The figure shows three views and two pictorial views of one solid part (mm, origin at its lowest corner). Answer the questions. Round coordinates to 2 decimals unless told otherwise and drop trailing zeros. Order: outer loops, then holes, each group sorted by start corner. A loop starts at its lowest first (then second) coordinate and runs counter-clockwise, first axis right, second up. Notation, with made-up numbers: (5, 13.25) - (31, 13.25) arc R33 ccw to (31, 50.25) - close; hole circle Ø7 at (87, 20). An arc over 180 degrees is marked (long way). Answer as a JSON object with one key per item and string values. Group by question number.
Q1. A cutting plane is placed at A-A on x = 10. Determine the outline of the cut face in (y, z), and give its area (3 significant figures).
Q2. A cutting plane is placed at C-C on y = 1. Determine the outline of the cut face in (x, z), and give its area (3 significant figures).
Q3. Consider line 1 (Z direction, x = 10, y = 2.5); line 2 (X direction, y = 5.5, z = 11) (1 decimal); line 3 (X direction, y = 2, z = 10) (1 decimal). Determine where each line is inside the solid, lowest interval first.
Q4. A cutting plane is placed at B-B on z = 12.5. Determine the outline of the cut face in (x, y), and give its area (3 significant figures).
Q5. Given pin 1 Ø3 at (x, z) = (72.5, 36.5) entering from +Y (1 decimal), flat-ended and moving along its own axis, determine where the tip first touches the part or whether it passes through.
Q6. A cutting plane is placed at D-D on x = 69.5. Determine the outline of the cut face in (y, z) (1 decimal), and give its area (3 significant figures).
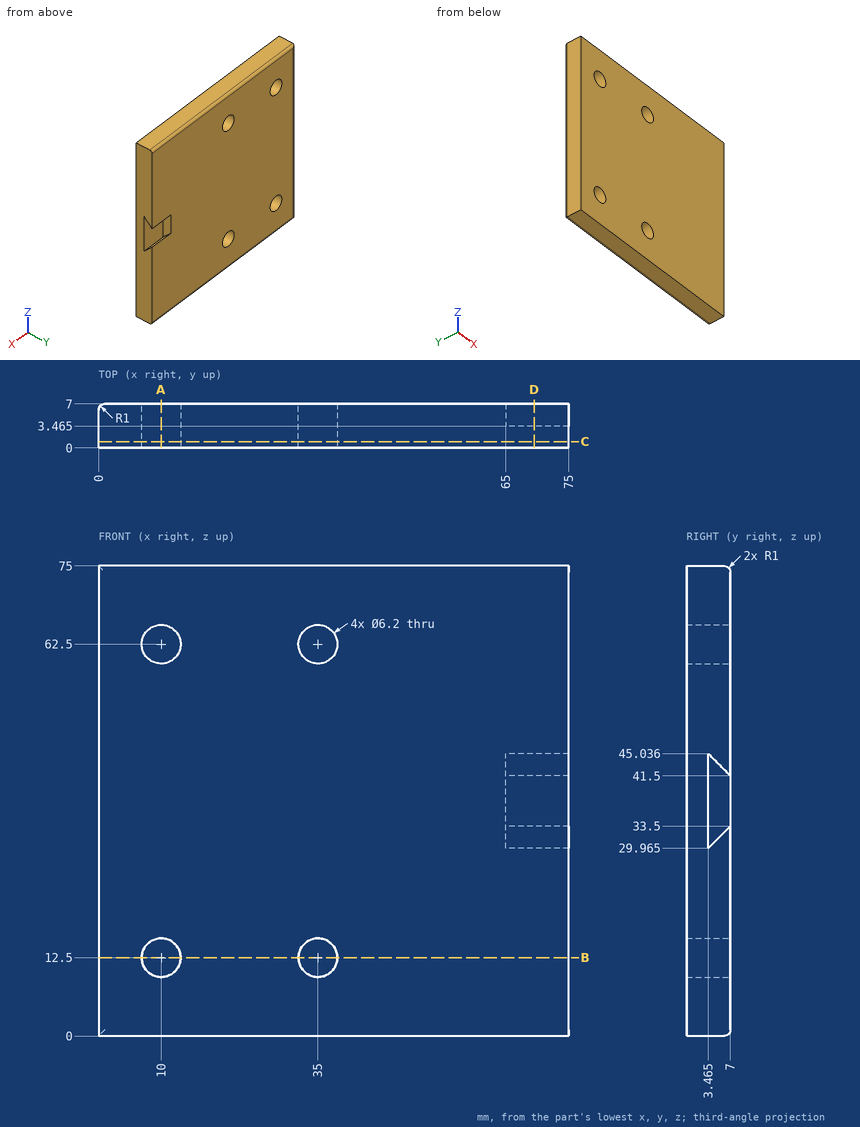
Result set:
{
 "1": {"outline": "(0, 0) - (6, 0) arc R1 ccw to (7, 1) - (7, 9.4) - (0, 9.4) - close; (0, 15.6) - (7, 15.6) - (7, 59.4) - (0, 59.4) - close; (0, 65.6) - (7, 65.6) - (7, 74) arc R1 ccw to (6, 75) - (0, 75) - close", "area": "438 mm²"},
 "2": {"outline": "(0, 0) - (75, 0) - (75, 75) - (0, 75) - close; hole circle Ø6.2 at (10, 12.5); hole circle Ø6.2 at (10, 62.5); hole circle Ø6.2 at (35, 12.5); hole circle Ø6.2 at (35, 62.5)", "area": "5,500 mm²"},
 "3": {"line 1": "z = 0 to 9.4, 15.6 to 59.4, 65.6 to 75", "line 2": "x = 0 to 7.3, 12.7 to 32.3, 37.7 to 75", "line 3": "x = 0 to 8.2, 11.8 to 33.2, 36.8 to 75"},
 "4": {"outline": "(0, 0) - (6.9, 0) - (6.9, 7) - (1, 7) arc R1 ccw to (0, 6) - close; (13.1, 0) - (31.9, 0) - (31.9, 7) - (13.1, 7) - close; (38.1, 0) - (75, 0) - (75, 7) - (38.1, 7) - close", "area": "438 mm²"},
 "5": {"pin 1": "stops at y = 3.5"},
 "6": {"outline": "(0, 0) - (6, 0) arc R1 ccw to (7, 1) - (7, 33.5) - (3.5, 30) - (3.5, 45) - (7, 41.5) - (7, 74) arc R1 ccw to (6, 75) - (0, 75) - close", "area": "484 mm²"}
}
